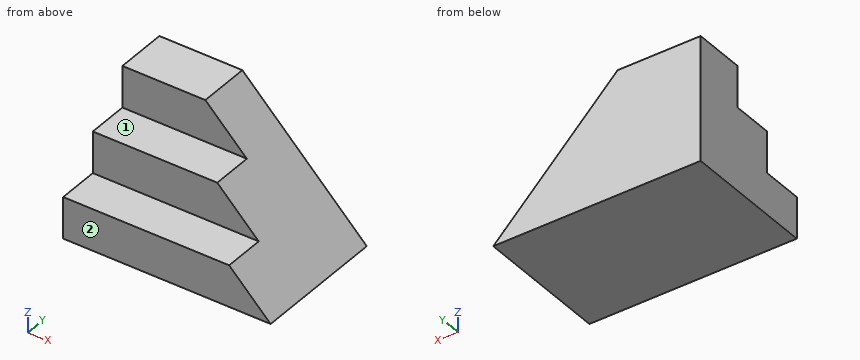
```python
from build123d import *

# Parameters (mm, degrees)
F0_W     = 100
F0_H     = 20
F1_DEPTH = 25
F2_DEPTH = 20
F3_DEPTH = 40
F4_SIZE  = 59.99999


# Not quite as in the source:
# - a fillet or chamfer is up to 0.001 mm smaller than in the source, because OpenCascade refuses the exact size


with BuildPart() as f1:
    # F0 (on Front) → F1 (new body)
    with BuildSketch(Plane.XZ):
        with Locations((50, 10)):
            Rectangle(F0_W, F0_H)
        with Locations((50, 30)):
            Rectangle(F0_W, F0_H)
        with Locations((50, 50)):
            Rectangle(F0_W, F0_H)
    extrude(amount=-F1_DEPTH)

    # F0 (on Front) → F2 (join)
    with BuildSketch(Plane.XZ):
        with Locations((50, 30)):
            Rectangle(F0_W, F0_H)
        with Locations((50, 10)):
            Rectangle(F0_W, F0_H)
    extrude(amount=F2_DEPTH)

    # F0 (on Front) → F3 (join)
    with BuildSketch(Plane.XZ):
        with Locations((50, 10)):
            Rectangle(F0_W, F0_H)
    extrude(amount=F3_DEPTH)

    # F4 (size 60 in the source; OpenCascade refuses exactly that, so slightly less here)
    f4_edges = [f1.edges().sort_by_distance(p)[0] for p in [
        (100, 12.5, 60),
    ]]
    chamfer(f4_edges, length=F4_SIZE)


solid = f1.part
```
Design review of the part built by this model. Coordinates are the model's own, in mm. Face numbers are marked on the shaded views. A direction names the side the tool comes from. Coordinates: 2 decimals unless noted, no trailing zeros. Order: outer loops, then holes, each group sorted by start corner. A loop starts at its lowest first (then second) coordinate and runs counter-clockwise, first axis right, second up. Notation, with made-up numbers: M 5,-39.75 L 55,-39.75 A15 cw 55,-25.75 Z; hole C 7,43 d3. An arc over 180 degrees is marked long. Answer as a JSON object with one key per item and string values. Group by question number.
1) Tool access review of the marked faces 1 and 2: name each direction out of +Z, -Z, +X, -X, +Y, -Y from which nothing blocks a thin tool from reaching the whole face with its end or side.
2) For pin 1 (3 mm diameter, centred on x = 15, y = -6, fed in from +Z); pin 2 (3 mm diameter, centred on x = 36, y = -23.5, fed in from +Z); pin 3 (1 mm diameter, centred on y = -14.5, z = 16, fed in from +X), all flat-tipped, find the tip position at first contact; note any pin that passes through.
3) Add section D-D, the plane x = 33.5. Write out the cut boundary in (y, z), then the cut area to 3 significant figures.
4) Add section C-C, the plane z = 24. Write out the cut boundary in (x, y).
5) Add section A-A, the plane x = 48. Write out the cut boundary in (y, z), then the cut area to 3 significant figures.
6) Wall thickness on L1, parallel to Y at x = 69.5, z = 29; L2, parallel to Z at x = 11, y = -24; L3, parallel to X at y = -18.5, z = 20.5: over which ranges is each line inside the solid? List them lowest first.
Computed values:
{
 "1": {"face 1": "+Z, +X, -X, -Y", "face 2": "+Z, -Z, +X, -X, -Y"},
 "2": {"pin 1": "stops at z = 40", "pin 2": "stops at z = 20", "pin 3": "stops at x = 84.5"},
 "3": {"outline": "M -40,0 L 25,0 L 25,60 L 0,60 L 0,40 L -20,40 L -20,20 L -40,20 Z", "area": "2,700 mm^2"},
 "4": {"outline": "M 0,-20 L 76,-20 L 76,25 L 0,25 Z"},
 "5": {"outline": "M -40,0 L 25,0 L 25,52 L 0,52 L 0,40 L -20,40 L -20,20 L -40,20 Z", "area": "2,500 mm^2"},
 "6": {"L1": "y = -20 to 25", "L2": "z = 0 to 20", "L3": "x = 0 to 79.5"}
}
